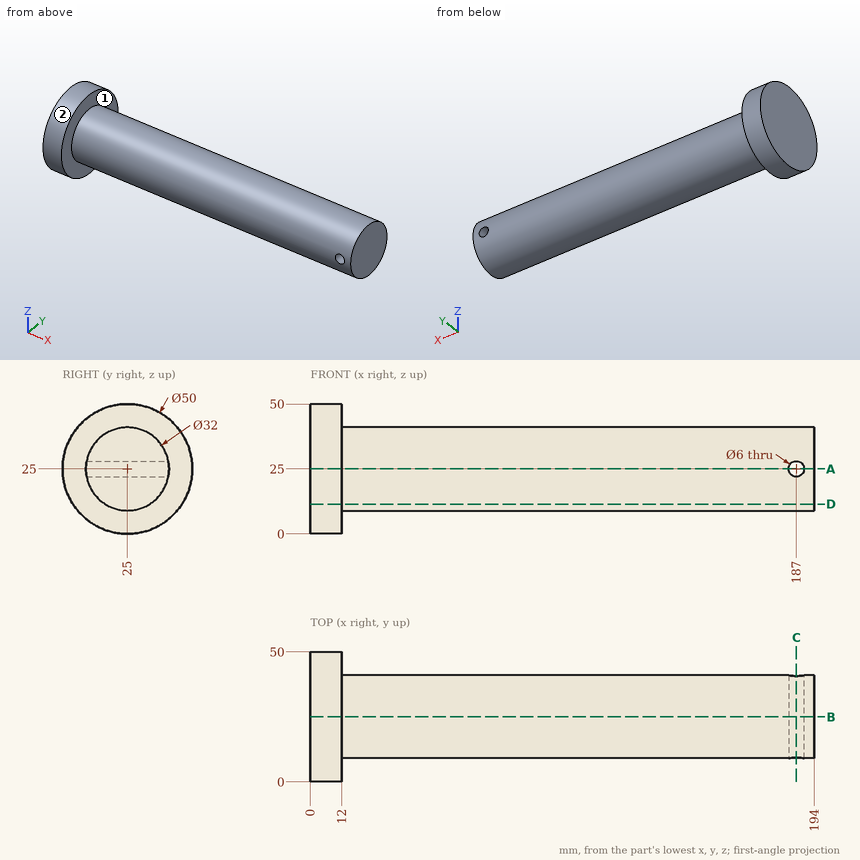
Study the drawing (mm; zero at the part's minimum x, y, z) and answer. A direction names the side the tool comes from. Give positions to 0.01 mm unless a question says otherwise; leave off trailing zeros. Loops run counter-clockwise (first coordinate to the right, second up) from the corner with the lowest first, then second, coordinate; pieces in that order, holes last. Notation, with made-up numbers: (-6.75, 36) - (24.25, 36) arc R18 ccw to (24.25, 69) - close; hole circle Ø2 at (-23, 83.25). An arc over 180 degrees is marked (long way). Answer in a Markdown table with one row per item. Add a question column.
Q1. The part is cut by section B-B (y = 25). Determine the outline of the cut face in (x, z).
Q2. The part is cut by section A-A (z = 25). Determine the outline of the cut face in (x, y).
Q3. A tool of negligible diameter and unlimited length cuts with its end or side. For the marked faces 1 and 2, from which of +Z, -Z, +X, -X, +Y, -Y can it reach the whole face along a straight path? Write none if from no direction.
Q4. The part is cut by section C-C (x = 187). Determine the outline of the cut face in (y, z).
Q5. Consider line 1 along X through (y, z) = (33, 25); line 2 along Z through (x, y) = (26, 25.5); line 3 along X through (y, z) = (2.5, 34.5). Determine where each line is inside the solid, lowest interval first.
Q6. The part is cut by section D-D (z = 11.5). Determine the outline of the cut face in (x, y), and give its area (3 significant figures).
Q7. Each of these flat-tipped pins is pushed along its axis until it touches: P1, Ø5.5, axis at x = 187, z = 25, coming from the -Y side; P2, Ø2, axis at x = 82, z = 31, coming from the +Y side; P3, Ø5, axis at x = 144.5, y = 21.5, coming from the -Z side; P4, Ø6, axis at x = 31, y = 29, coming from the +Z side. Where does it stop, or does it pass through?
Solution:
| question | item | result |
|---|---|---|
| 1 | outline | (0, 0) - (12, 0) - (12, 9) - (194, 9) - (194, 41) - (12, 41) - (12, 50) - (0, 50) - close; hole circle Ø6 at (187, 25) |
| 2 | outline | (0, 0) - (12, 0) - (12, 9) - (184, 9) - (184, 41) - (12, 41) - (12, 50) - (0, 50) - close; (190, 9) - (194, 9) - (194, 41) - (190, 41) - close |
| 3 | face 1 | +X |
| 3 | face 2 | +X, -X |
| 4 | outline | (9.28, 22) arc R16 ccw to (40.72, 22) - close; (9.28, 28) - (40.72, 28) arc R16 ccw to start |
| 5 | line 1 | x = 0 to 184, 190 to 194 |
| 5 | line 2 | z = 9.01 to 40.99 |
| 5 | line 3 | x = 0 to 12 |
| 6 | outline | (0, 3.96) - (12, 3.96) - (12, 16.41) - (194, 16.41) - (194, 33.59) - (12, 33.59) - (12, 46.04) - (0, 46.04) - close |
| 6 | area | 3,630 mm² |
| 7 | P1 | passes through |
| 7 | P2 | stops at y = 40.2 |
| 7 | P3 | stops at z = 9.03 |
| 7 | P4 | stops at z = 40.97 |
